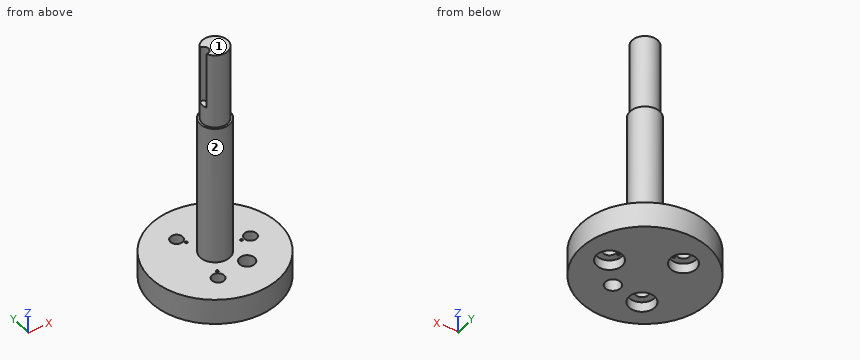
Autodesk Inventor part; units mm, degrees
ref_plane "YZ Plane" through (0, 0, 0) normal (1, 0, 0) x (0, 1, 0)
ref_plane "XZ Plane" through (0, 0, 0) normal (0, 1, 0) x (-1, 0, 0)
ref_plane "XY Plane" through (0, 0, 0) normal (0, 0, 1) x (1, 0, 0)
sketch "Sketch1" plane through (0, 0, 0) normal (0, 0, 1) x (1, 0, 0)
  circle A0 centre (0, 0) radius 12.7
  dimension "d0" = 25.4
extrude "Extrusion1" add sketch "Sketch1" along normal blind 48.26
sketch "Sketch2" plane through (0, 0, 48.26) normal (0, 0, 1) x (1, 0, 0)
  circle A0 centre (0, 0) radius 12.7
  circle A1 centre (0, 0) radius 2.9464
  dimension "d3" = 5.8928
extrude "Extrusion2" cut sketch "Sketch2" against normal blind 43.18
sketch "Sketch3" plane through (0, 0, 0) normal (0, 0, -1) x (-1, 0, 0)
  circle A0 centre (-7, 0) radius 0.847
  circle A1 centre (3.5, 6.0622) radius 0.847
  arc A2 (5.3333, -1.3437) -> (5.3333, 1.3437) centre (6, 0) ccw
  circle A3 centre (3.5, -6.0622) radius 0.847
  circle A4 centre (6, 0) radius 1.5
hole "Hole1" at (7, 0, 0) at (-3.5, -6.0622, 0) at (-3.5, 6.0622, 0) direction (0, 0, 1) diameter 2.4384 end through all counterbore diameter 5.08 counterbore depth 2
sketch "Sketch4" plane through (0, 0, 0) normal (0, 0, -1) x (-1, 0, 0)
  circle A0 centre (0, 0) radius 12.7
  line L0 (0, 0) -> (-2.921, -5.0593)
  line L1 (0, -17.78) -> (0, 17.78)
  line L2 (17.78, 0) -> (-17.78, 0)
  dimension "d37" = 60
  dimension "d38" = 5.842
hole "Hole2" at (2.921, -5.0593, 0) direction (0, 0, 1) diameter 2.9972 end through all
sketch "Sketch5" plane through (0, 0, 5.08) normal (0, 0, 1) x (1, 0, 0)
  circle A0 centre (-3.5, 6.0622) radius 1.2192
  circle A1 centre (-3.5, -6.0622) radius 1.2192
  circle A2 centre (7, 0) radius 1.2192
  circle A3 centre (0, 0) radius 2.9464
  circle A4 centre (0, 0) radius 12.7
  circle A5 centre (2.921, -5.0593) radius 1.4986
ref_plane "Top Ref" through (0, 0, 37.4401) normal (0, 0, 1) x (1, 0, 0)
ref_plane "Bottom Ref" through (0, 0, 15.08) normal (0, 0, 1) x (1, 0, 0)
ref_plane "Work Plane4" through (0, 0, 33.6301) normal (0, 0, 1) x (1, 0, 0)
ref_plane "Work Plane5" through (0, 0, 33.1221) normal (0, 0, 1) x (1, 0, 0)
ref_plane "Work Plane6" through (0, 0, 36.9321) normal (0, 0, 1) x (1, 0, 0)
sketch "Sketch6" plane through (0, 0, 48.26) normal (0, 0, 1) x (1, 0, 0)
  circle A0 centre (0, 0) radius 2.9464
  circle A1 centre (0, 0) radius 2.54
  dimension "d25" = 5.08
extrude "Extrusion3" cut sketch "Sketch6" against normal up to surface (15.1379 mm away)
sketch "Sketch7" plane through (0, 0, 48.26) normal (0, 0, 1) x (1, 0, 0)
  circle A0 centre (0, 0) radius 2.54
  circle A1 centre (-2.286, 0) radius 1.016
  dimension "d28" = 2.032
  dimension "d29" = 2.286
hole "Hole3" at (-2.286, 0, 48.26) direction (0, 0, -1) diameter 2.032 depth 11.3279
sketch "Sketch8" plane through (0, 0, 0) normal (0, 0, -1) x (-1, 0, 0)
  circle A0 centre (0, 0) radius 12.7
  point P0 (-5.2324, 0)
  dimension "d42" = 5.2324
hole "Hole4" at (5.2324, 0, 0) direction (0, 0, 1) diameter 0.508 end through all
pattern_circular "Circular Pattern1" count 3 over 360 about axis through (0, 0, -10) along (0, 0, 1) of "Hole4"
properties part number "Jig_TopHeightAligner"
Could you check a few things on this model? Use its own coordinates, in mm. Face numbers are marked on the shaded views. A direction names the side the tool comes from. Give positions to 0.01 mm unless a question says otherwise; leave off trailing zeros. Order: outer loops, then holes, each group sorted by start corner. A loop starts at its lowest first (then second) coordinate and runs counter-clockwise, first axis right, second up. Notation, with made-up numbers: (17.5, 47) - (25.5, 47) arc R22 ccw to (25.5, 62) - close; hole circle Ø10 at (43.5, -25.75). An arc over 180 degrees is marked (long way). Return JSON: item names as keys, results as strings. Group by question number.
Q1. Which directions (+Z, -Z, +X, -X, +Y, -Y) give clear straight access to the entire face, cutting with the end or side of a thin tool? Please do the marked faces 1 and 2.
Q2. Please list where these lines run through material, in increasing order: line 1 along Y through (x, z) = (-3.5, 2.9); line 2 along Z through (x, y) = (7.5, 9.5); line 3 along Y through (x, z) = (0, 42). Write a range as [from, to].
Q3. Suppose I cut it at A-A, the plane x = 0. Please give me the cut outline in (y, z), and give its area (3 significant figures).
Q4. Will these pins go through, and if not, where does the flat tip stop? pin 1 Ø2 at (x, y) = (7, 0) entering from -Z; pin 2 Ø5 at (x, z) = (4, 14.5) entering from +Y; pin 3 Ø6 at (x, y) = (-3.5, 6.06) entering from +Z; pin 4 Ø2.5 at (x, y) = (-4, -5) entering from -Z.
Q5. Suppose I cut it at B-B, the plane x = -3.5. Please give me the cut outline in (y, z).
Q6. Suppose I cut it at C-C, the plane z = 34.5. Please give me the cut outline in (x, y).
Q7. Suppose I cut it at D-D, the plane x = 3.5. Please give me the cut outline in (y, z), and give its area (3 significant figures).
Resolved:
{
 "1": {"face 1": "+Z, +X, -X, +Y, -Y", "face 2": "+Z"},
 "2": {"line 1": "y = [-12.21, -7.28], [-4.84, 4.84], [7.28, 12.21]", "line 2": "z = [0, 5.08]", "line 3": "y = [-2.54, 2.54]"},
 "3": {"outline": "(-12.7, 0) - (12.7, 0) - (12.7, 5.08) - (2.95, 5.08) - (2.95, 33.12) - (2.54, 33.12) - (2.54, 48.26) - (-2.54, 48.26) - (-2.54, 33.12) - (-2.95, 33.12) - (-2.95, 5.08) - (-12.7, 5.08) - close", "area": "371 mm2"},
 "4": {"pin 1": "passes through", "pin 2": "stops at y = 2.54", "pin 3": "stops at z = 5.08", "pin 4": "stops at z = 2"},
 "5": {"outline": "(-12.21, 0) - (-8.6, 0) - (-8.6, 2) - (-7.28, 2) - (-7.28, 5.08) - (-12.21, 5.08) - close; (-4.84, 2) - (-3.52, 2) - (-3.52, 0) - (3.52, 0) - (3.52, 2) - (4.84, 2) - (4.84, 5.08) - (-4.84, 5.08) - close; (7.28, 2) - (8.6, 2) - (8.6, 0) - (12.21, 0) - (12.21, 5.08) - (7.28, 5.08) - close"},
 "6": {"outline": "circle Ø5.08 at (0, 0)"},
 "7": {"outline": "(-12.21, 0) - (-6.44, 0) - (-6.44, 5.08) - (-12.21, 5.08) - close; (-3.68, 0) - (12.21, 0) - (12.21, 5.08) - (-3.68, 5.08) - close", "area": "110 mm2"}
}
